Input: part model. Units: mm. Frame: model coordinates. A direction names the side the tool comes from. Round coordinates to 2 decimals unless told otherwise and drop trailing zeros. Loops run counter-clockwise (first coordinate to the right, second up) from the corner with the lowest first, then second, coordinate; pieces in that order, holes last.
(1) Access query for faces 4 (the face through (-2, 16, -70)), 5 (the face through (-54, 10, -6)), 6 (the face through (0, 15, -42)), 7 (the face through (18, 30, -46)). Directions: +Z, -Z, +X, -X, +Y, -Y. A direction counts if a zero-diameter tool reaches every point of the face in a straight line with its end or side. Return the directions, or none.
(2) First-contact query: pin 1 Ø2 at (x, z) = (-18.5, -46.5) entering from -Y; pin 2 Ø0.8 at (y, z) = (10, -46.5) entering from +X; pin 3 Ø0.8 at (x, z) = (16, -46) entering from -Y. Flat tips, straight axial feed; report the tip coordinate or a pass-through.
(3) Cut plane D-D, the plane y = 26. Output: boundary loops of the cut face in (x, z) (3 decimals).
(4) Cut plane A-A, the plane y = 15. Output: boundary loops of the cut face in (x, z), and give its area (3 significant figures).
(5) Cut plane C-C, the plane z = -55. Output: boundary loops of the cut face in (x, y).
(6) Cut plane B-B, the plane x = -45. Output: boundary loops of the cut face in (y, z), and give its area (3 significant figures).
(7) Line query: line 1 (Z direction, x = -13.5, y = 56.5); line 2 (Y direction, x = -37, z = -35); line 3 (Y direction, x = 14, z = -54). Output: solid intervals per line, ascending.
(8) Draft query along Y for faces 1 (the face through (-55, 25, 0)), 2 (the face through (27.988, 13.901, -57.325)), 3 (the face through (18, 0, -46)). Return one class per face: released by +Y, released by -Y, zero draft, split by the parting line, or undercut.
Solid Edge part; units mm, degrees
sketch "Sketch1" plane through (0, 0, 0) normal (0, -1, 0) x (1, 0, 0)
  line L0 (-40, 0) -> (-70, 0)
  arc A0 (-70, 0) -> (0, -70) centre (0, 0) ccw
  line L1 (0, -40) -> (0, -70)
  arc A1 (-40, 0) -> (0, -40) centre (0, 0) ccw
extrude "Protrusion1" add sketch "Sketch1" against normal blind 30
sketch "Sketch2" plane through (-55, 15, 0) normal (0, 0, 1) x (1, 0, 0)
  line L0 (15, 5) -> (-15, 5)
  line L1 (-15, 5) -> (-15, -5)
  line L2 (-15, -5) -> (15, -5)
extrude "ExtrudedCutout_1" cut sketch "Sketch2" along normal mid plane 24 material side at (-55, 19.95, 0)
sketch "Sketch3" plane through (0, 0, -45) normal (0, 0, 1) x (1, 0, 0)
  arc A0 (-22, 65) -> (-22, -35) centre (-22, 15) cw
  line L0 (-22, 65) -> (-22, -35)
extrude "ExtrudedProtrusion_2" add sketch "Sketch3" against normal blind 25
sketch "Sketch4" plane through (0, 0, -45) normal (0, 0, 1) x (1, 0, 0)
  line L0 (25.697, 0) -> (10, 0)
  line L1 (10, 30) -> (10, 0)
  line L2 (10, 30) -> (25.697, 30)
extrude "ExtrudedCutout_2" cut sketch "Sketch4" along normal mid plane 5 material side at (17.8485, 0.05, -45)
Reported:
1. face 4: -Z, +X, -X, +Y, -Y
1. face 5: +Z, +X, -X
1. face 6: +Z, +X, +Y, -Y
1. face 7: +Z, +X
2. pin 1: stops at y = -34.94
2. pin 2: stops at x = 10
2. pin 3: stops at y = -17.96
3. outline: (-70, 0) arc R70 ccw to (-22, -66.453) - (-22, -70) - (26.775, -70) - (26.775, -47.5) - (10, -47.5) - (10, -45) - (0, -45) - (0, -40) arc R40 cw to (-40, 0) - close
4. outline: (-68.96, -12) arc R70 ccw to (-22, -66.45) - (-22, -70) - (28, -70) - (28, -47.5) - (10, -47.5) - (10, -45) - (0, -45) - (0, -40) arc R40 cw to (-38.16, -12) - close
4. area: 2,910 mm2
5. outline: (-43.3, 0) - (-22, 0) - (-22, -35) arc R50 ccw to (-22, 65) - (-22, 30) - (-43.3, 30) - close
6. outline: (0, -53.62) - (30, -53.62) - (30, 0) - (20, 0) - (20, -12) - (10, -12) - (10, 0) - (0, 0) - close
6. area: 1,490 mm2
7. line 1: z = -70 to -45
7. line 2: y = 0 to 30
7. line 3: y = -19.7 to 49.7
8. face 1: zero draft
8. face 2: split by the parting line
8. face 3: undercut
